Work out the finished part from the listing and answer in its coordinate system (mm). Round coordinates to 2 decimals unless told otherwise and drop trailing zeros. Loops run counter-clockwise (first coordinate to the right, second up) from the corner with the lowest first, then second, coordinate; pieces in that order, holes last. Notation, with made-up numbers: (-25.5, 66.5) - (12.5, 66.5) arc R14 ccw to (12.5, 74.5) - close; hole circle Ø7 at (85.5, 22.5). An arc over 180 degrees is marked (long way). Return JSON: item names as keys, results as strings.
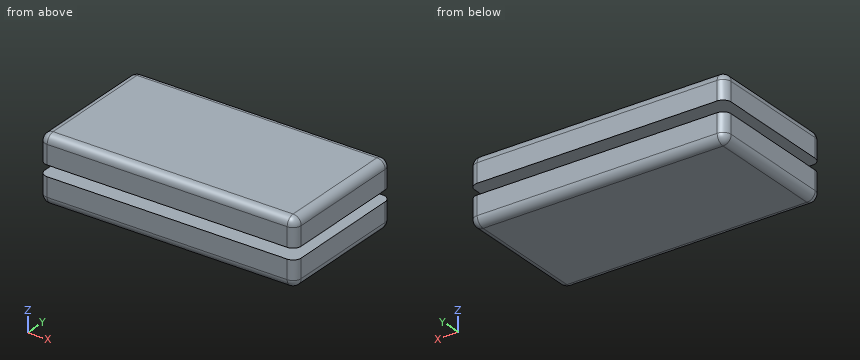
Autodesk Fusion 360 part; units mm, degrees
sketch "Sketch1" plane through (0, 0, 0) normal (0, 0, 1) x (1, 0, 0)
  line L0 (0, 0) -> (23.5, 0)
  line L1 (0, 0) -> (0, -12.25)
  line L2 (0, -12.25) -> (23.5, -12.25)
  line L3 (23.5, 0) -> (23.5, -12.25)
  line L4 (0, 0) -> (5.5, 0)
  line L5 (23.5, -12.25) -> (18, -12.25)
  line L6 (18, -10) -> (5.5, -10)
  line L7 (5.5, -10) -> (5.5, -2.25)
  line L8 (5.5, -2.25) -> (18, -2.25)
  line L9 (18, -2.25) -> (18, -10)
  dimension "d1" = 23.5
  dimension "d2" = 12.25
  dimension "d3" = 5.5
  dimension "d4" = 2.25
  dimension "d5" = 5.5
  dimension "d6" = 2.25
extrude "Extrude1" add sketch "Sketch1" along normal blind 6 contours L6 L7 L8 L9 makes body 1
extrude "Extrude2" add sketch "Sketch1" along normal blind 6 separate body makes body 2
sketch "Sketch2" plane through (23.5, 0, 0) normal (1, 0, 0) x (0, 1, 0)
  line L0 (-12.25, 0) -> (0, 0)
  line L1 (0, 0) -> (0, 6)
  line L2 (0, 6) -> (-12.25, 6)
  line L3 (-12.25, 6) -> (-12.25, 0)
  line L4 (0, 3.5) -> (-2.25, 3.5)
  line L5 (-12.25, 2.5) -> (-10, 2.5)
  line L6 (-12.25, 2.5) -> (0, 2.5)
  line L7 (0, 2.5) -> (0, 3.5)
  line L8 (0, 3.5) -> (-12.25, 3.5)
  line L9 (-12.25, 3.5) -> (-12.25, 2.5)
  dimension "d12" = 2.25
  dimension "d13" = 2.5
  dimension "d14" = 2.25
extrude "Extrude3" cut sketch "Sketch2" against normal blind 29 contours L1 L3 L4 L5 L6 L7 L8 L9 bodies 1 2 makes body 4 at (1.8333, -4.8333, 3.5) makes body 3 at (9.6667, -4.8333, 3.5)
extrude "Extrude4" add 1 faces at (13.8333, -7.4167, 2.5) along direction (0, 0, 1) blind 2 on bodies 1 bodies 1 2 3 4
fillet "Fillet1" radius 0.75 16 edges at (0, 0, 4.75) (11.75, 0, 6) (0, -6.125, 6) (11.75, -12.25, 6) (0, -12.25, 4.75) (23.5, -12.25, 4.75) (23.5, -6.125, 6) (23.5, 0, 4.75) (11.75, 0, 0) (0, 0, 1.25) (0, -6.125, 0) (0, -12.25, 1.25) (11.75, -12.25, 0) (23.5, -12.25, 1.25) (23.5, -6.125, 0) (23.5, 0, 1.25) on bodies 1
1) Flat-ended cylindrical pins translate along their axes: pin 1 (1.5 mm diameter, centred on y = -6.5, z = 4, fed in from -X); pin 2 (0.5 mm diameter, centred on y = -5.5, z = 3, fed in from +X); pin 3 (0.8 mm diameter, centred on x = 10.5, z = 3, fed in from -Y). Find the tip coordinate at first contact, or state that the pin passes through.
Verdict:
{"pin 1": "stops at x = 0", "pin 2": "stops at x = 18", "pin 3": "stops at y = -10"}
2) Section D-D (y = -7.5) is taken. Give the vertices of the cut face in (x, z).
Verdict:
{"outline": "(0, 0.75) arc R0.75 ccw to (0.75, 0) - (22.75, 0) arc R0.75 ccw to (23.5, 0.75) - (23.5, 2.5) - (18, 2.5) - (18, 3.5) - (23.5, 3.5) - (23.5, 5.25) arc R0.75 ccw to (22.75, 6) - (0.75, 6) arc R0.75 ccw to (0, 5.25) - (0, 3.5) - (5.5, 3.5) - (5.5, 2.5) - (0, 2.5) - close"}
3) Section C-C (x = 7) is taken. Give the vertices of the cut face in (y, z), and give its area (3 significant figures).
Verdict:
{"outline": "(-12.25, 0.75) arc R0.75 ccw to (-11.5, 0) - (-0.75, 0) arc R0.75 ccw to (0, 0.75) - (0, 2.5) - (-2.25, 2.5) - (-2.25, 3.5) - (0, 3.5) - (0, 5.25) arc R0.75 ccw to (-0.75, 6) - (-11.5, 6) arc R0.75 ccw to (-12.25, 5.25) - (-12.25, 3.5) - (-10, 3.5) - (-10, 2.5) - (-12.25, 2.5) - close", "area": "68.5 mm2"}
4) Find the intervals of material crossed by L1, parallel to Z at x = 1.75, y = -4.5; L2, parallel to X at y = -4.25, z = 3; L3, parallel to Y at x = 8.75, z = 5.3, in increasing order.
Verdict:
{"L1": "z = 0 to 2.5, 3.5 to 6", "L2": "x = 5.5 to 18", "L3": "y = -12.25 to 0"}
5) Section B-B (x = 21.5) is taken. Give the vertices of the cut face in (y, z), and give its area (3 significant figures).
Verdict:
{"outline": "(-12.25, 0.75) arc R0.75 ccw to (-11.5, 0) - (-0.75, 0) arc R0.75 ccw to (0, 0.75) - (0, 2.5) - (-12.25, 2.5) - close; (-12.25, 3.5) - (0, 3.5) - (0, 5.25) arc R0.75 ccw to (-0.75, 6) - (-11.5, 6) arc R0.75 ccw to (-12.25, 5.25) - close", "area": "60.8 mm2"}
6) Section A-A (y = -1) is taken. Give the vertices of the cut face in (x, z), and give its area (3 significant figures).
Verdict:
{"outline": "(0, 0.75) arc R0.75 ccw to (0.75, 0) - (22.75, 0) arc R0.75 ccw to (23.5, 0.75) - (23.5, 2.5) - (0, 2.5) - close; (0, 3.5) - (23.5, 3.5) - (23.5, 5.25) arc R0.75 ccw to (22.75, 6) - (0.75, 6) arc R0.75 ccw to (0, 5.25) - close", "area": "117 mm2"}
